Part model, mm, in its own coordinate system. Face numbers are marked on the shaded views. A direction names the side the tool comes from. Round coordinates to 2 decimals unless told otherwise and drop trailing zeros. Write each loop counter-clockwise with the first axis right and the second up, starting at its lowest first coordinate (ties: lowest second). Pieces come first, ordered by that corner, then holes. Notation, with made-up numbers: (80, 48) -> (87, 48) arc R26 cw to (87, 67) -> close; hole circle Ø11 at (-30, 59). An arc over 180 degrees is marked (long way). Return JSON: item names as keys, results as strings. Group by question number.
(1) Mould opens along X. For the marked faces 1, 2 and 3 say: +X half, -X half, draft (parallel to the pull), parting line (faces both ways), or undercut.
(2) Saw through at B-B (x = 60.5). List the corners of the cut face in (y, z), plus the area to 3 significant figures.
(3) Tool access for the marked faces 4, 5 and 6: list every direction of +Z, -Z, +X, -X, +Y, -Y with a clear straight run to the whole face (end or side of a thin tool).
(4) Drill centre lines: L1, parallel to Z at x = 17, y = 21; L2, parallel to X at y = 98.5, z = -2; L3, parallel to Y at x = 118, z = -63. Where is each one in solid material? Low to high. Write a range as from..to.
(5) Saw through at D-D (z = -13). List the corners of the cut face in (x, y).
(6) Saw through at C-C (x = -35.5). List the corners of the cut face in (y, z), plus the area to 3 significant figures.
(7) Drop flat-ended pins along their axis: pin 1 Ø2 at (x, y) = (-14.5, 98.5) entering from -Z; pin 2 Ø1.9 at (x, z) = (-10, -65.5) entering from +Y; pin 3 Ø1.2 at (x, y) = (147, 39) entering from -Z. Give the stop position or say it passes through.
(8) Saw through at A-A (z = 56.5). List the corners of the cut face in (x, y).
from build123d import *

# Parameters (mm, degrees)
SKETCH_1_W          = 238
SKETCH_1_H          = 140
EXTRUDE_3_DEPTH     = 125
SHELL_1_T           = -4
SKETCH_2_W          = 230
SKETCH_2_H          = 80
CUT_EXTRUDE_1_DEPTH = 120
SKETCH_5_W          = 4
SKETCH_5_H          = 117
EXTRUDE_6_DEPTH     = 1.5
SKETCH_6_W          = 4
SKETCH_6_H          = 117
EXTRUDE_7_DEPTH     = 1.5
EXTRUDE_8_DEPTH     = 5
EXTRUDE_9_DEPTH     = 230
EXTRUDE_10_DEPTH    = 227
SKETCH_10_W         = 2.5
SKETCH_10_H         = 74.5
EXTRUDE_11_DEPTH    = 1.5
SKETCH_11_W         = 2.5
SKETCH_11_H         = 74.5
EXTRUDE_12_DEPTH    = 1.5
SKETCH_12_W         = 4
SKETCH_12_H         = 111
EXTRUDE_14_DEPTH    = 1.5
SKETCH_13_W         = 2
SKETCH_13_H         = 111
SKETCH_13_W_2       = 4
EXTRUDE_17_DEPTH    = 1.5
SKETCH_14_W         = 28
SKETCH_14_H         = 48
CUT_EXTRUDE_3_DEPTH = 18
SKETCH_15_W         = 30
SKETCH_15_H         = 22
CUT_EXTRUDE_4_DEPTH = 18
SKETCH_16_W         = 2
SKETCH_16_H         = 111
EXTRUDE_18_DEPTH    = 1.5
SKETCH_17_W         = 4
SKETCH_17_H         = 111
EXTRUDE_19_DEPTH    = 1.5
SKETCH_19_W         = 4
SKETCH_19_H         = 111
EXTRUDE_20_DEPTH    = 1.5
SKETCH_20_W         = 4
SKETCH_20_H         = 111
EXTRUDE_21_DEPTH    = 1.5


with BuildPart() as part:
    # 草图1 → 凸台-拉伸3 (new body)
    with BuildSketch(Plane(origin=(0, 0, 0), x_dir=(1, 0, 0), z_dir=(0, 1, 0))):
        with Locations((32.875338753, -3.224932249)):
            Rectangle(SKETCH_1_W, SKETCH_1_H)
    extrude(amount=EXTRUDE_3_DEPTH)

    # 抽壳1
    shell_1_openings = [part.faces().sort_by_distance(p)[0] for p in [
        (32.875338753, 125, 3.224932249),
    ]]
    offset(amount=SHELL_1_T, openings=shell_1_openings, kind=Kind.INTERSECTION)

    # 草图2 → 切除-拉伸1 (cut)
    with BuildSketch(Plane.XY.offset(-62.775067751)):
        with Locations((32.875338753, 85)):
            Rectangle(SKETCH_2_W, SKETCH_2_H)
    extrude(amount=-CUT_EXTRUDE_1_DEPTH, mode=Mode.SUBTRACT)

    # 草图5 → 凸台-拉伸6 (add)
    with BuildSketch(Plane.ZY.offset(-147.875338753)):
        with Locations((-60.775067751, 62.5)):
            Rectangle(SKETCH_5_W, SKETCH_5_H)
    extrude(amount=EXTRUDE_6_DEPTH)

    # 草图6 → 凸台-拉伸7 (add)
    with BuildSketch(Plane(origin=(-82.124661247, 0, 0), x_dir=(0, 0, -1), z_dir=(1, 0, 0))):
        with Locations((60.775067751, 62.5)):
            Rectangle(SKETCH_6_W, SKETCH_6_H)
    extrude(amount=EXTRUDE_7_DEPTH)

    # 草图7 → 凸台-拉伸8 (add)
    with BuildSketch(Plane(origin=(0, 0, -66.775067751), x_dir=(-1, 0, 0), z_dir=(0, 0, -1))):
        Polygon((-151.875338753, 125), (-147.875338753, 125), (-147.875338753, 4), (82.124661247, 4), (82.124661247, 125), (86.124661247, 125), (86.124661247, 0), (-151.875338753, 0), align=None)
    extrude(amount=EXTRUDE_8_DEPTH)

    # 草图8 → 凸台-拉伸9 (add)
    with BuildSketch(Plane.ZY.offset(-147.875338753)):
        Polygon((-66.645720039, 46.5), (-66.775067751, 37.387932584), (-69.145720039, 45), (-69.145720039, 46.5), align=None)
    extrude(amount=EXTRUDE_9_DEPTH)

    # 草图9 → 凸台-拉伸10 (add)
    with BuildSketch(Plane.ZY.offset(-146.375338753)):
        Polygon((-62.775067751, 46.5), (-58.775067751, 46.5), (-58.775067751, 44.5), (-62.775067751, 43), align=None)
    extrude(amount=EXTRUDE_10_DEPTH)

    # 草图10 → 凸台-拉伸11 (add)
    with BuildSketch(Plane.ZY.offset(-147.875338753)):
        with Locations((-67.895720039, 83.75)):
            Rectangle(SKETCH_10_W, SKETCH_10_H)
    extrude(amount=EXTRUDE_11_DEPTH)

    # 草图11 → 凸台-拉伸12 (add)
    with BuildSketch(Plane(origin=(-82.124661247, 0, 0), x_dir=(0, 0, -1), z_dir=(1, 0, 0))):
        with Locations((67.895720039, 83.75)):
            Rectangle(SKETCH_11_W, SKETCH_11_H)
    extrude(amount=EXTRUDE_12_DEPTH)

    # 草图12 → 凸台-拉伸14 (add)
    with BuildSketch(Plane.ZY.offset(-147.875338753)):
        with Locations((36.224932249, 59.5)):
            Rectangle(SKETCH_12_W, SKETCH_12_H)
        with Locations((29.024932249, 59.5)):
            Rectangle(SKETCH_12_W, SKETCH_12_H)
    extrude(amount=EXTRUDE_14_DEPTH)

    # 草图13 → 凸台-拉伸17 (add)
    with BuildSketch(Plane.ZY.offset(-147.875338753)):
        with Locations((68.224932249, 59.5)):
            Rectangle(SKETCH_13_W, SKETCH_13_H)
        with Locations((62.224932249, 59.5)):
            Rectangle(SKETCH_13_W_2, SKETCH_13_H)
    extrude(amount=EXTRUDE_17_DEPTH)

    # 草图14 → 切除-拉伸3 (cut)
    with BuildSketch(Plane.ZY.offset(-146.375338753)):
        with Locations((50.224932249, 46.5)):
            Rectangle(SKETCH_14_W, SKETCH_14_H)
    extrude(amount=-CUT_EXTRUDE_3_DEPTH, mode=Mode.SUBTRACT)

    # 草图15 → 切除-拉伸4 (cut)
    with BuildSketch(Plane(origin=(0, 0, -66.775067751), x_dir=(-1, 0, 0), z_dir=(0, 0, -1))):
        with Locations((-117.875338753, 20.693966292)):
            Rectangle(SKETCH_15_W, SKETCH_15_H)
        with Locations((-72.875338753, 20.693966292)):
            Rectangle(SKETCH_15_W, SKETCH_15_H)
    extrude(amount=-CUT_EXTRUDE_4_DEPTH, mode=Mode.SUBTRACT)

    # 草图16 → 凸台-拉伸18 (add)
    with BuildSketch(Plane(origin=(-82.124661247, 0, 0), x_dir=(0, 0, -1), z_dir=(1, 0, 0))):
        with Locations((-68.224932249, 59.5)):
            Rectangle(SKETCH_16_W, SKETCH_16_H)
    extrude(amount=EXTRUDE_18_DEPTH)

    # 草图17 → 凸台-拉伸19 (add)
    with BuildSketch(Plane(origin=(-82.124661247, 0, 0), x_dir=(0, 0, -1), z_dir=(1, 0, 0))):
        with Locations((-62.224932249, 59.5)):
            Rectangle(SKETCH_17_W, SKETCH_17_H)
    extrude(amount=EXTRUDE_19_DEPTH)

    # 草图19 → 凸台-拉伸20 (add)
    with BuildSketch(Plane(origin=(-82.124661247, 0, 0), x_dir=(0, 0, -1), z_dir=(1, 0, 0))):
        with Locations((-36.224932249, 59.5)):
            Rectangle(SKETCH_19_W, SKETCH_19_H)
    extrude(amount=EXTRUDE_20_DEPTH)

    # 草图20 → 凸台-拉伸21 (add)
    with BuildSketch(Plane(origin=(-82.124661247, 0, 0), x_dir=(0, 0, -1), z_dir=(1, 0, 0))):
        with Locations((-29.024932249, 59.5)):
            Rectangle(SKETCH_20_W, SKETCH_20_H)
    extrude(amount=EXTRUDE_21_DEPTH)


solid = part.part
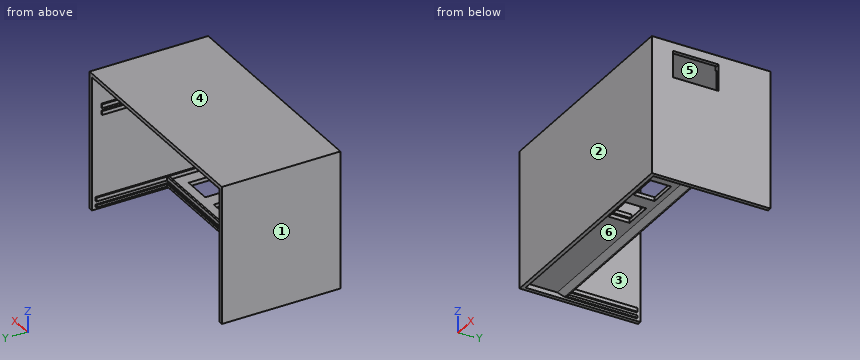
Computed values:
{
 "1": {"face 1": "-X half", "face 2": "draft", "face 3": "undercut"},
 "2": {"outline": "(0, -71.78) -> (4, -71.78) -> (4, -66.78) -> (9.69, -66.78) -> (9.69, -62.78) -> (4, -62.78) -> (4, 69.22) -> (125, 69.22) -> (125, 73.22) -> (0, 73.22) -> close; (31.69, -66.78) -> (37.39, -66.78) -> (45, -69.15) -> (46.5, -69.15) -> (46.5, -66.65) -> (45, -66.67) -> (45, -62.78) -> (46.5, -62.78) -> (46.5, -58.78) -> (44.5, -58.78) -> (43, -62.78) -> (31.69, -62.78) -> close", "area": "1,160 mm2"},
 "3": {"face 4": "+Z, +X, -X, +Y, -Y", "face 5": "+Y", "face 6": "-Z"},
 "4": {"L1": "-66.78..-62.78, 69.22..73.22", "L2": "-86.12..-82.12, 147.88..151.88", "L3": "0..9.69, 31.69..45"},
 "5": {"outline": "(-86.12, 0) -> (151.88, 0) -> (151.88, 125) -> (147.88, 125) -> (147.88, 4) -> (-82.12, 4) -> (-82.12, 125) -> (-86.12, 125) -> close"},
 "6": {"outline": "(0, -71.78) -> (4, -71.78) -> (4, -66.78) -> (37.39, -66.78) -> (45, -69.15) -> (46.5, -69.15) -> (46.5, -66.65) -> (45, -66.67) -> (45, -62.78) -> (46.5, -62.78) -> (46.5, -58.78) -> (44.5, -58.78) -> (43, -62.78) -> (4, -62.78) -> (4, 69.22) -> (125, 69.22) -> (125, 73.22) -> (0, 73.22) -> close", "area": "1,250 mm2"},
 "7": {"pin 1": "z = 69.22", "pin 2": "y = 45", "pin 3": "z = -67.46"},
 "8": {"outline": "(-86.12, 0) -> (151.88, 0) -> (151.88, 22.5) -> (147.88, 22.5) -> (147.88, 4) -> (-82.12, 4) -> (-82.12, 125) -> (-86.12, 125) -> close; (147.88, 70.5) -> (151.88, 70.5) -> (151.88, 125) -> (147.88, 125) -> close"}
}
